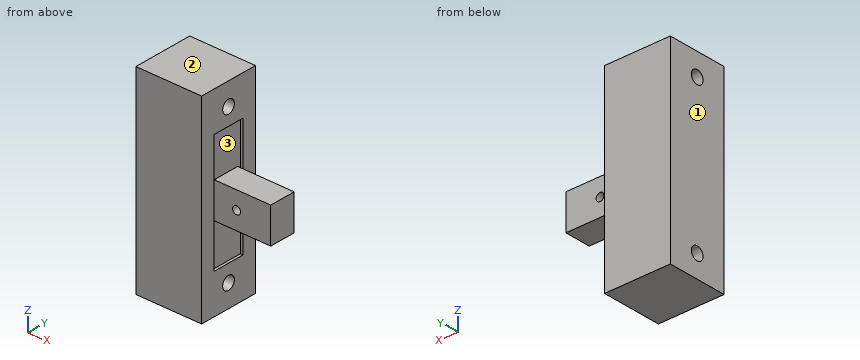
```python
from build123d import *

# Parameters (mm, degrees)
SKETCH_1_W          = 10
SKETCH_1_H          = 30
EXTRUDE_1_DEPTH     = 4.6
SKETCH_2_W          = 18
SKETCH_2_H          = 5
CUT_EXTRUDE_1_DEPTH = 0.4
SKETCH_3_W          = 5.4
SKETCH_3_H          = 4
EXTRUDE_2_DEPTH     = 8.6
SKETCH_4_R          = 0.6
CUT_EXTRUDE_2_DEPTH = 4
SKETCH_5_R          = 1
CUT_EXTRUDE_3_DEPTH = 11


with BuildPart() as part:
    # 草图1 → 凸台-拉伸1 (new body, symmetric)
    with BuildSketch(Plane(origin=(0, 0, 0), x_dir=(1, 0, 0), z_dir=(0, 1, 0))):
        Rectangle(SKETCH_1_W, SKETCH_1_H)
    extrude(amount=EXTRUDE_1_DEPTH, both=True)

    # 草图2 → 切除-拉伸1 (cut)
    with BuildSketch(Plane(origin=(5, 0, 0), x_dir=(0, 0, -1), z_dir=(1, 0, 0))):
        Rectangle(SKETCH_2_W, SKETCH_2_H)
    extrude(amount=-CUT_EXTRUDE_1_DEPTH, mode=Mode.SUBTRACT)

    # 草图3 → 凸台-拉伸2 (add)
    with BuildSketch(Plane(origin=(4.6, 0, 0), x_dir=(0, 0, -1), z_dir=(1, 0, 0))):
        Rectangle(SKETCH_3_W, SKETCH_3_H)
    extrude(amount=EXTRUDE_2_DEPTH)

    # 草图4 → 切除-拉伸2 (cut)
    with BuildSketch(Plane(origin=(0, 2, 0), x_dir=(1, 0, 0), z_dir=(0, 1, 0))):
        with Locations((8, 0)):
            Circle(SKETCH_4_R)
    extrude(amount=-CUT_EXTRUDE_2_DEPTH, mode=Mode.SUBTRACT)

    # 草图5 → 切除-拉伸3 (cut, through all)
    with BuildSketch(Plane(origin=(5, 0, 0), x_dir=(0, 0, -1), z_dir=(1, 0, 0))):
        with Locations((11.6, 0)):
            Circle(SKETCH_5_R)
        with Locations((-11.6, 0)):
            Circle(SKETCH_5_R)
    extrude(amount=-CUT_EXTRUDE_3_DEPTH, mode=Mode.SUBTRACT)


solid = part.part
```
The model under review builds one solid part; all positions refer to its coordinate system, in mm. Face numbers are marked on the shaded views. Round coordinates to 2 decimals unless told otherwise and drop trailing zeros. Loops run counter-clockwise (first coordinate to the right, second up) from the corner with the lowest first, then second, coordinate; pieces in that order, holes last. Notation, with made-up numbers: (-25.5, 62.5) - (-5.5, 62.5) arc R27 ccw to (-5.5, 95.5) - close; hole circle Ø6 at (-37.5, 72.25). An arc over 180 degrees is marked (long way). Write each question's results on one line, items separated by ' | '. Start each with the question number.
Q1. Insertion check: P1, Ø2.5, axis at y = 0, z = 11.6, coming from the +X side; P2, Ø10, axis at x = 11, z = -7, coming from the -Y side; P3, Ø2, axis at x = 11, y = 0.5, coming from the -Z side. Each pin has a flat end and moves straight along its axis. Give the tip position at first contact, or say it passes through.
Q2. Take a section at B-B on z = -11.6. Give the boundary of the cut face in (x, y), plus the area to 3 significant figures.
Q3. Wall thickness on line 1 along Y through (x, z) = (1.5, -11.6); line 2 along Z through (x, y) = (8, 0.65); line 3 along X through (y, z) = (-0.05, 0): over which ranges is each line inside the solid? List them lowest first. Write a range as [from, to].
Q4. Take a section at C-C on x = 8. Give the boundary of the cut face in (y, z).
Q5. Take a section at A-A on y = 0. Give the boundary of the cut face in (x, z), plus the area to 3 significant figures.
Q6. Take a section at D-D on x = 1. Give the boundary of the cut face in (y, z).
Q7. Draft analysis for pull direction Z (two halves, no side actions). For the marked faces 1, 2 and 3, state which applies: pulls with the +Z half, pulls with the -Z half, needs draft (parallel to the pull), parting line crosses it, or undercut.
Data:
1) P1: stops at x = 5 | P2: stops at y = -2 | P3: stops at z = -2.7
2) outline: (-5, -4.6) - (5, -4.6) - (5, -1) - (-5, -1) - close; (-5, 1) - (5, 1) - (5, 4.6) - (-5, 4.6) - close | area: 72.0 mm²
3) line 1: y = [-4.6, -1], [1, 4.6] | line 2: z = [-2.7, -0.6], [0.6, 2.7] | line 3: x = [-5, 7.4], [8.6, 13.2]
4) outline: (-2, -2.7) - (2, -2.7) - (2, -0.6) - (-2, -0.6) - close; (-2, 0.6) - (2, 0.6) - (2, 2.7) - (-2, 2.7) - close
5) outline: (-5, -15) - (5, -15) - (5, -12.6) - (-5, -12.6) - close; (-5, -10.6) - (5, -10.6) - (5, -9) - (4.6, -9) - (4.6, -2.7) - (13.2, -2.7) - (13.2, 2.7) - (4.6, 2.7) - (4.6, 9) - (5, 9) - (5, 10.6) - (-5, 10.6) - close; (-5, 12.6) - (5, 12.6) - (5, 15) - (-5, 15) - close; hole circle Ø1.2 at (8, 0) | area: 298 mm²
6) outline: (-4.6, -15) - (4.6, -15) - (4.6, 15) - (-4.6, 15) - close; hole circle Ø2 at (0, -11.6); hole circle Ø2 at (0, 11.6)
7) face 1: needs draft | face 2: pulls with the +Z half | face 3: undercut
